Model file for the job. Use its own axes, mm. A direction names the side the tool comes from. Give positions to 0.01 mm unless a question says otherwise; leave off trailing zeros. Write each loop counter-clockwise with the first axis right and the second up, starting at its lowest first coordinate (ties: lowest second). Pieces come first, ordered by that corner, then holes.
```python
from build123d import *

# Parameters (mm, degrees)
F2_SIZE = 0.25


with BuildPart() as f1:
    # F0 (on Top) → F1 (revolve)
    with BuildSketch(Plane.XY):
        Polygon((0, -5.8332120482), (-29, -5.8332120482), (-29, -10.3332120482), (-25.5, -10.3332120482), (-25.5, -9.3332120482), (-24.4, -9.3332120482), (-24.4, -10.3332120482), (-4.6, -10.3332120482), (-4.6, -9.3332120482), (-3.5, -9.3332120482), (-3.5, -10.3332120482), (0, -10.3332120482), align=None)
    revolve(axis=Axis((-14.5, -0.8332120482, 0), (-1, 0, 0)))

    # F2
    f2_edges = [f1.edges().sort_by_distance(p)[0] for p in [
        (0, 8.666788, 0),
        (-29, 8.666788, 0),
        (-29, 4.166788, 0),
        (0, 4.166788, 0),
    ]]
    chamfer(f2_edges, length=F2_SIZE)


solid = f1.part
```
1. Which spindle directions (+Z, -Z, +X, -X, +Y, -Y) get a long thin tool onto all of the face, cutting with end or side? Do faces 1 (the flat face through (0, -5, -4)), 2 (the flat face through (-3.5, -8, -5)). Say none if no direction does.
Calculated:
face 1: +Z, -Z, +X, +Y, -Y
face 2: none
2. Pull direction Y, two halves, no side cores. Call faces 3 (the cylindrical face through (-27.102, 1.226, -9.274)), 4 (the cylindrical face through (-14.7, 0.25, -4.88)), 5 (the flat face through (-29, 3, -4)): +Y half, -Y half, draft (parallel to the pull), parting line (faces both ways), or undercut.
Calculated:
face 3: parting line
face 4: undercut
face 5: draft
3. Pin check, flat tips, straight feed: P1, Ø8, axis at x = -15, z = -6.5, coming from the +Y side; P2, Ø3, axis at x = -11, z = -4.5, coming from the +Y side; P3, Ø2, axis at x = -12, z = 4.5, coming from the -Y side (3 decimals). Stop position of each tip, or through.
Calculated:
P1: stops at y = 8.33
P2: stops at y = 8.18
P3: stops at y = -9.665
4. Probe probe 1 along X at (y, z) = (-4, 8); probe 2 along Y at (x, z) = (-25.75, 1.5); probe 3 along Z at (x, y) = (-18, -8.75). List the from-to ranges inside material, lowest first.
Calculated:
probe 1: x = -29 to -25.5, -24.4 to -4.6, -3.5 to 0
probe 2: y = -10.21 to -5.6, 3.94 to 8.55
probe 3: z = -5.25 to 5.25
5. Slice it at A-A, the plane x = -12. Write the cut outline in (y, z).
Calculated:
outline: circle Ø19 at (-0.83, 0); hole circle Ø10 at (-0.83, 0)
